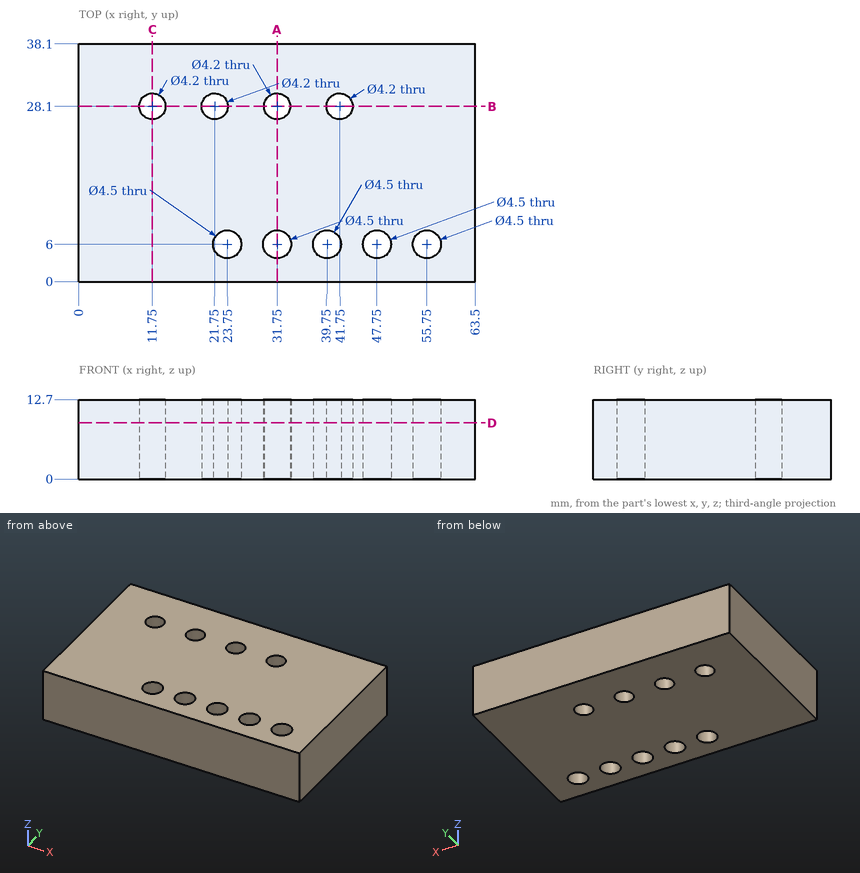
Study the drawing (mm; zero at the part's minimum x, y, z) and answer. Coordinates: 2 decimals unless noted, no trailing zeros. Write each loop counter-clockwise with the first axis right and the second up, starting at its lowest first coordinate (ties: lowest second). Pieces come first, ordered by that corner, then holes. Notation, with made-up numbers: M 30,26.25 L 47,26.25 A20 ccw 47,64.25 Z; hole C 63,7.25 d11. An arc over 180 degrees is marked long. Use a Markdown table: item, result. Add a question column.
1. Straight lines are drawn through the part: line 1 along Y through (x, z) = (31.75, 9.5); line 2 along Y through (x, z) = (11.75, 8.25); line 3 along Y through (x, z) = (47.75, 4.25). For each, find the intervals that lie inside material, in ascending order. Write a range as [from, to].
2. Section B-B (y = 28.1) is taken. Give the vertices of the cut face in (x, z), plus the area to 3 significant figures.
3. Given P1, Ø5, axis at x = 23.75, y = 6, coming from the +Z side, flat-ended and moving along its own axis, determine where the tip first touches the part or whether it passes through.
4. Section D-D (z = 9) is taken. Count the separate pieces of the cut face and the enclosed holes in it, plus the area to 3 significant figures.
5. Section A-A (x = 31.75) is taken. Give the vertices of the cut face in (y, z).
6. Section C-C (x = 11.75) is taken. Give the vertices of the cut face in (y, z).
Data:
| question | item | result |
|---|---|---|
| 1 | line 1 | y = [0, 3.75], [8.25, 26], [30.2, 38.1] |
| 1 | line 2 | y = [0, 26], [30.2, 38.1] |
| 1 | line 3 | y = [0, 3.75], [8.25, 38.1] |
| 2 | outline | M 0,0 L 9.65,0 L 9.65,12.7 L 0,12.7 Z; M 13.85,0 L 19.65,0 L 19.65,12.7 L 13.85,12.7 Z; M 23.85,0 L 29.65,0 L 29.65,12.7 L 23.85,12.7 Z; M 33.85,0 L 39.65,0 L 39.65,12.7 L 33.85,12.7 Z; M 43.85,0 L 63.5,0 L 63.5,12.7 L 43.85,12.7 Z |
| 2 | area | 593 mm2 |
| 3 | P1 | stops at z = 12.7 |
| 4 | separate pieces | 1 |
| 4 | enclosed holes | 9 |
| 4 | area | 2,280 mm2 |
| 5 | outline | M 0,0 L 3.75,0 L 3.75,12.7 L 0,12.7 Z; M 8.25,0 L 26,0 L 26,12.7 L 8.25,12.7 Z; M 30.2,0 L 38.1,0 L 38.1,12.7 L 30.2,12.7 Z |
| 6 | outline | M 0,0 L 26,0 L 26,12.7 L 0,12.7 Z; M 30.2,0 L 38.1,0 L 38.1,12.7 L 30.2,12.7 Z |
